Verification items for the finished model (mm, model axes). Face numbers are marked on the shaded views. A direction names the side the tool comes from. Round coordinates to 2 decimals unless told otherwise and drop trailing zeros. Loops run counter-clockwise (first coordinate to the right, second up) from the corner with the lowest first, then second, coordinate; pieces in that order, holes last. Notation, with made-up numbers: M -8,51 L 5,51 A17 cw 5,84 Z; hole C 42,-13 d2. An arc over 180 degrees is marked long. One line per item, written item: value.
from build123d import *

# Parameters (mm, degrees)
SKETCH_1_R          = 16
EXTRUDE_1_DEPTH     = 20.6
EXTRUDE_2_DEPTH     = 3
SKETCH_3_R          = 3
EXTRUDE_3_DEPTH     = 16.3
CUT_EXTRUDE_START   = -12
CUT_EXTRUDE_1_DEPTH = 12
CUT_EXTRUDE_START_2 = -4.3
SKETCH_7_R          = 3
CUT_EXTRUDE_2_DEPTH = 4.3


with BuildPart() as part:
    # ｽｹｯﾁ1 → ﾎﾞｽ - 押し出し1 (new body)
    with BuildSketch(Plane.XY):
        with Locations(Location((0, 0, 0), (0, 0, 180))):
            Circle(SKETCH_1_R)
    extrude(amount=EXTRUDE_1_DEPTH)

    # ｽｹｯﾁ2 → ﾎﾞｽ - 押し出し2 (add)
    with BuildSketch(Plane.XY.offset(20.6)):
        with BuildLine():
            Line((-9, 4.358898944), (-9, -4.358898944))
            ThreePointArc((-9, -4.358898944), (0, -10), (9, -4.358898944))
            Line((9, -4.358898944), (9, 4.358898944))
            ThreePointArc((9, 4.358898944), (0, 10), (-9, 4.358898944))
        make_face()
    extrude(amount=EXTRUDE_2_DEPTH)

    # ｽｹｯﾁ3 → ﾎﾞｽ - 押し出し3 (add)
    with BuildSketch(Plane.XY.offset(23.6)):
        Circle(SKETCH_3_R)
    extrude(amount=EXTRUDE_3_DEPTH)

    # ｽｹｯﾁ4 → ｶｯﾄ - 押し出し1 (cut)
    with BuildSketch(Plane.XY.offset(39.9).offset(CUT_EXTRUDE_START)):
        with BuildLine():
            Line((-2.236067977, 2), (2.236067977, 2))
            ThreePointArc((2.236067977, 2), (0, 3), (-2.236067977, 2))
        make_face()
    extrude(amount=CUT_EXTRUDE_1_DEPTH, mode=Mode.SUBTRACT)

    # ｽｹｯﾁ7 → ｶｯﾄ - 押し出し2 (cut)
    with BuildSketch(Plane.XY.offset(39.9).offset(CUT_EXTRUDE_START_2)):
        with Locations(Location((0, 0, 0), (0, 0, 138.189685104))):
            Circle(SKETCH_7_R)
    extrude(amount=CUT_EXTRUDE_2_DEPTH, mode=Mode.SUBTRACT)


solid = part.part
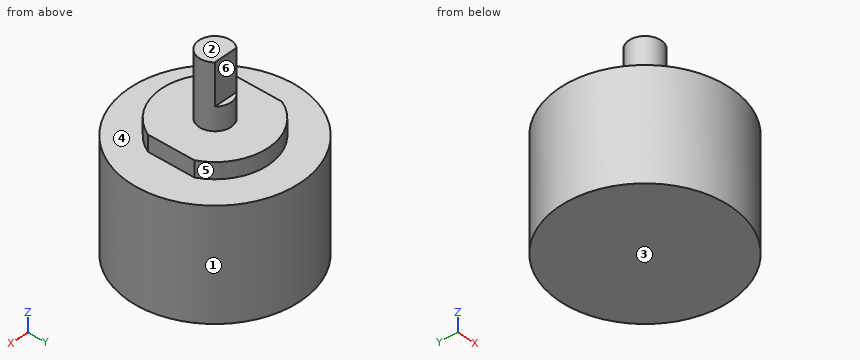
(1) Tool access check on the marked faces 3, 4, 5 and 6. Record the directions out of +Z, -Z, +X, -X, +Y, -Y that give a thin tool (end or side, any length) a straight path to the whole face; none if there is none.
Completed:
face 3: -Z, +X, -X, +Y, -Y
face 4: +Z
face 5: +Z, +Y
face 6: +Z, +X, -X, +Y
(2) Thickness scan on L1, parallel to Z at x = -0.5, y = 11; L2, parallel to Y at x = 0.5, z = 12.5; L3, parallel to Z at x = -8, y = 1.5. Record the ranges inside material, lowest first. Write a range as from..to.
Completed:
L1: z = 0..20.6
L2: y = -15.99..15.99
L3: z = 0..23.6
(3) Sectioned sample at C-C on z = 13. Enter the section's corners in (x, y).
Completed:
outline: C 0,0 d32
(4) Mould release check, pull along X, two halves, no side actions. Record for the marked faces 1 and 2: +X half, -X half, draft (parallel to the pull), parting line (faces both ways), or undercut.
Completed:
face 1: parting line
face 2: draft
(5) Sectioned sample at A-A on x = 0. Enter the section's corners in (y, z).
Completed:
outline: M -16,0 L 16,0 L 16,20.6 L 10,20.6 L 10,23.6 L 3,23.6 L 3,27.9 L 2,27.9 L 2,35.6 L -3,35.6 L -3,23.6 L -10,23.6 L -10,20.6 L -16,20.6 Z
(6) Sectioned sample at B-B on y = 0. Enter the section's corners in (x, z), and give its area (3 significant figures).
Completed:
outline: M -16,0 L 16,0 L 16,20.6 L 9,20.6 L 9,23.6 L 3,23.6 L 3,35.6 L -3,35.6 L -3,23.6 L -9,23.6 L -9,20.6 L -16,20.6 Z
area: 785 mm^2
(7) Sectioned sample at D-D on x = 5. Enter the section's corners in (y, z).
Completed:
outline: M -15.2,0 L 15.2,0 L 15.2,20.6 L 8.66,20.6 L 8.66,23.6 L -8.66,23.6 L -8.66,20.6 L -15.2,20.6 Z
(8) Depth check by flat-ended pin: pin 1 Ø12 at (x, z) = (1, 27.5) entering from -Y; pin 2 Ø1.5 at (y, z) = (-1, 13.5) entering from +X; pin 3 Ø1.5 at (x, y) = (-1.5, -6) entering from +Z. Enter the tip coordinate at first touch or a pass-through.
Completed:
pin 1: stops at y = -10
pin 2: stops at x = 16
pin 3: stops at z = 23.6
